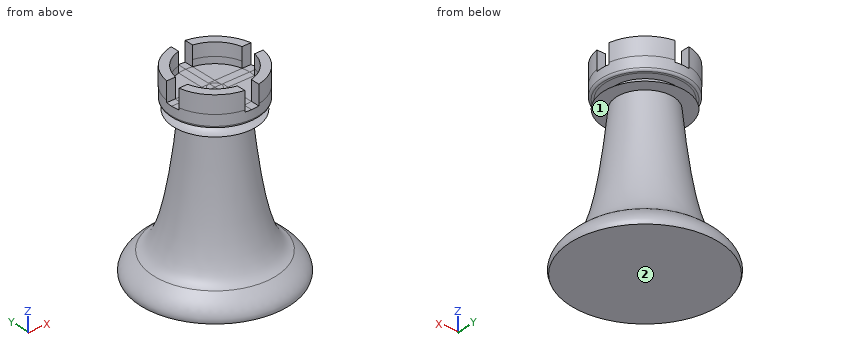
Autodesk Fusion 360 part; units mm, degrees
sketch "Tura" plane through (0, 0, 0) normal (0, 1, 0) x (1, 0, 0)
  line L0 (0, 0) -> (17, 0)
  line L1 (0, 0) -> (0, -38.5138)
  line L2 (0, -38.5138) -> (0, -35)
  line L3 (0, -38.5138) -> (0, -35)
  line L4 (0, 0) -> (0, -5)
  line L5 (14, -5) -> (0, -5)
  spline S0 degree 5 poles (6.5259, -34) (6.6855, -32.318) (7.0209, -29.0147) (7.5725, -24.2418) (8.412, -18.2671) (9.7194, -11.7648) (11.1016, -7.8229) (12.4226, -5.9311) (13.4497, -5.2188) (14, -5) knots 0 0 0 0 0 0 0.2 0.4 0.6 0.8 1 1 1 1 1 1
  line L6 (12.8092, -5.4735) -> (15.1908, -4.5265)
  spline S1 degree 5 poles (14, -5) (14.3724, -4.7164) (15.065, -4.1591) (15.9469, -3.3525) (16.8041, -2.3367) (17.2264, -1.3701) (17.2496, -0.692) (17.1232, -0.2556) (17.015, -0.0297) (17, 0) knots 0 0 0 0 0 0 0.1 0.2 0.3 0.4 0.415205 0.415205 0.415205 0.415205 0.415205 0.415205
  line L7 (17.1967, -0.3896) -> (16.8033, 0.3896)
  line L8 (0, -37.3622) -> (0, -38.5138)
  line L9 (0, -36) -> (9, -36)
  line L10 (0, -38) -> (0, -36)
  line L11 (8, -40) -> (8, -43)
  line L12 (8, -43) -> (10, -43)
  line L13 (10, -43) -> (10, -36.5)
  line L14 (9.5, -36) -> (9, -36)
  line L15 (0, -36) -> (9.5003, -36)
  line L16 (9.5, -34) -> (0, -34)
  line L17 (0, -34) -> (0, -36)
  arc A0 (9.5005, -34) -> (9.5, -34) centre (9.5, -36.5) ccw
  arc A1 (9.5003, -36) -> (9.5005, -34) centre (9.5003, -35) ccw
  arc A2 (10, -36.5) -> (9.5, -36) centre (9.5, -36.5) ccw
  line L18 (-1.7845, -43) -> (1.4873, -43)
  line L19 (1.4873, -43) -> (1.4873, -38.5138)
  line L20 (1.4873, -38.5138) -> (-1.7845, -38.5138)
  line L21 (-1.7845, -38.5138) -> (-1.7845, -43)
  line L22 (1.4873, -38.5138) -> (8, -38.5138)
  line L23 (8, -38.5138) -> (8, -40)
  point P0 (10, -35)
  dimension "d1" = 17
  dimension "d3" = 10
  dimension "d5" = 3
  dimension "d6" = 2.5
  dimension "d7" = 1
  dimension "d8" = 0.5
revolve "Revolve2" add sketch "Tura" angle 360 about axis through (0, 0, 0) along (0, 0, 1) contours L0 L1 L4 L5 S1 | L1 L5 S0 L16 | L1 L2 L3 L9 L15 L16 L17 A0 | L1 L2 L3 L8 L9 L10 L11 L12 L13 L15 A0 L20 L22 L23 | L9 L13 L14 L15 A0 A2
extrude "Extrude2" cut sketch "Tura" along normal blind 10 contours L18 L19 L20 L21
pattern_circular "C-Pattern1" count 4 over 360 about axis through (0, 0, 0) along (0, 0, 1) of "Extrude2"
Part model, mm, in its own coordinate system. Face numbers are marked on the shaded views. A direction names the side the tool comes from. Give positions to 0.01 mm unless a question says otherwise; leave off trailing zeros. Use one line per item in the form item = value.
(1) Tool access for the marked faces 1 and 2: list every direction of +Z, -Z, +X, -X, +Y, -Y with a clear straight run to the whole face (end or side of a thin tool).
Solution:
face_1 = none
face_2 = -Z, +X, -X, +Y, -Y
(2) Flat gauge pins, fed straight in: P1, Ø0.5, axis at x = -9, y = -0.5, coming from the +Z side; P2, Ø6, axis at x = 11.5, z = 28, coming from the -Y side; P3, Ø0.6, axis at y = -9, z = 41, coming from the +X side; P4, Ø0.6, axis at y = 8.5, z = 40, coming from the -X side. Where does each tip first touch, or does it go through?
Solution:
P1 = 38.51
P2 = through
P3 = 4.93
P4 = -5.72
(3) Drill centre lines: line 1 (Z direction, x = -2, y = 5.5); line 2 (Y direction, x = 8.5, z = 41); line 3 (X direction, y = -1.5, z = 28). Where is each one in solid material? Low to high. Write a range as from..to.
Solution:
line_1 = 0..38.51
line_2 = -5.27..-1.49, 1.78..5.27
line_3 = -7..7
